Autodesk Inventor part; units mm, degrees
ref_plane "YZ Plane" through (0, 0, 0) normal (1, 0, 0) x (0, 1, 0)
ref_plane "XZ Plane" through (0, 0, 0) normal (0, 1, 0) x (-1, 0, 0)
ref_plane "XY Plane" through (0, 0, 0) normal (0, 0, 1) x (1, 0, 0)
sketch "Sketch1" plane through (0, 0, 0) normal (0, 0, 1) x (1, 0, 0)
  circle A0 centre (0, 0) radius 15
  circle A1 centre (0, 10.5) radius 2.25
  circle A2 centre (-7.4246, 7.4246) radius 2.25
  circle A3 centre (-10.5, 0) radius 2.25
  circle A4 centre (-7.4246, -7.4246) radius 2.25
  circle A5 centre (0, -10.5) radius 2.25
  circle A6 centre (7.4246, -7.4246) radius 2.25
  circle A7 centre (10.5, 0) radius 2.25
  circle A8 centre (7.4246, 7.4246) radius 2.25
  dimension "d0" = 30
  dimension "d2" = 4.5
  dimension "d5" = 360
extrude "Extrusion1" add sketch "Sketch1" along normal blind 5
sketch "Sketch2" plane through (0, 0, 5) normal (0, 0, 1) x (1, 0, 0)
  circle A0 centre (0, 0) radius 4
  circle A1 centre (0, 0) radius 5.3414
  circle A2 centre (0, 0) radius 6
  dimension "d9" = 8
extrude "Extrusion2" add sketch "Sketch2" along normal blind 5 contours A2
extrude "Extrusion3" add sketch "Sketch2" along normal blind 15 contours A1
extrude "Extrusion4" cut sketch "Sketch2" against normal blind 21 contours A0
properties part number "Hubnew"
Geometry check sheet. Reference: the model listing, model coordinates, mm. A direction names the side the tool comes from. Round coordinates to 2 decimals unless told otherwise and drop trailing zeros. Loops run counter-clockwise (first coordinate to the right, second up) from the corner with the lowest first, then second, coordinate; pieces in that order, holes last. Notation, with made-up numbers: (-7, 42) -> (13, 42) arc R30 cw to (13, 78) -> close; hole circle Ø5 at (-21, 14). An arc over 180 degrees is marked (long way). Use a Markdown table: item, result.
(1) Scan lines: probe 1 along Z at (x, y) = (-1.5, 6.75); probe 2 along Y at (x, z) = (0, 15); probe 3 along Y at (x, z) = (-2, 9.5). Record each from-to range of solid material in increasing order.
Calculated:
| item | result |
|---|---|
| probe 1 | 0 to 5 |
| probe 2 | -5.34 to -4, 4 to 5.34 |
| probe 3 | -5.66 to -3.46, 3.46 to 5.66 |
(2) Mould release check, pull along X, two halves, no side actions. Record for faces 3 (the flat face through (-0.2, -6.5, 5)), 4 (the cylindrical face through (8.463, -5.428, 2.465)), 5 (the cylindrical face through (-6.386, -5.428, 2.465)), 6 (the cylindrical face through (-14.985, -0.66, 2.465)): released by +X, released by -X, zero draft, split by the parting line, or undercut.
Calculated:
| item | result |
|---|---|
| face 3 | zero draft |
| face 4 | undercut |
| face 5 | undercut |
| face 6 | split by the parting line |
(3) Sectioned sample at C-C (z = 3.5). Give the number of separate pieces and of enclosed holes in the cut face, then the cut area to 3 significant figures.
Calculated:
| item | result |
|---|---|
| separate pieces | 1 |
| enclosed holes | 9 |
| area | 529 mm² |
(4) Sectioned sample at A-A (x = 0). Enter the section's corners in (y, z).
Calculated:
| item | result |
|---|---|
| outline | (-15, 0) -> (-12.75, 0) -> (-12.75, 5) -> (-15, 5) -> close; (-8.25, 0) -> (-4, 0) -> (-4, 20) -> (-5.34, 20) -> (-5.34, 10) -> (-6, 10) -> (-6, 5) -> (-8.25, 5) -> close; (4, 0) -> (8.25, 0) -> (8.25, 5) -> (6, 5) -> (6, 10) -> (5.34, 10) -> (5.34, 20) -> (4, 20) -> close; (12.75, 0) -> (15, 0) -> (15, 5) -> (12.75, 5) -> close |
(5) Sectioned sample at D-D (y = 10.5). Enter the section's corners in (x, z).
Calculated:
| item | result |
|---|---|
| outline | (-10.71, 0) -> (-2.25, 0) -> (-2.25, 5) -> (-10.71, 5) -> close; (2.25, 0) -> (10.71, 0) -> (10.71, 5) -> (2.25, 5) -> close |
(6) Set-up check for faces 1 (the flat face through (-4, -4, 10)), 2 (the flat face through (2, 4, 20)): record each of +Z, -Z, +X, -X, +Y, -Y from which the full face is reachable in a straight line by a thin tool's end or side.
Calculated:
| item | result |
|---|---|
| face 1 | +Z |
| face 2 | +Z, +X, -X, +Y, -Y |
(7) Go/stop test with flat-tipped pins: P1, Ø5, axis at y = -1.5, z = 15, coming from the +X side; P2, Ø5, axis at y = 3.5, z = 13.5, coming from the +X side; P3, Ø4, axis at x = -3.5, z = 2.5, coming from the -Y side. Record where each tip stops, or that it passes through.
Calculated:
| item | result |
|---|---|
| P1 | x = 5.34 |
| P2 | x = 5.25 |
| P3 | y = -14.92 |
